Build history of the part. All positions in model axes, mm. A direction names the side the tool comes from. Give positions to 0.01 mm unless a question says otherwise; leave off trailing zeros. Order: outer loops, then holes, each group sorted by start corner. A loop starts at its lowest first (then second) coordinate and runs counter-clockwise, first axis right, second up. Notation, with made-up numbers: (37, 40.5) - (69, 40.5) arc R26 ccw to (69, 56.5) - close; hole circle Ø6 at (-35, 37.25). An arc over 180 degrees is marked (long way). Use a Markdown table: item, result. Add a question column.
(1) Slice it at C-C (z = -0.75). Write the cut outline in (x, y).
(2) Slice it at B-B (z = 5). Write the cut outline in (x, y) (1 decimal), then the cut area to 3 significant figures.
(3) Slice it at D-D (z = 13). Write the cut outline in (x, y).
(4) Flat gauge pins, fed straight in: pin 1 (0.9 mm diameter, centred on x = -23.5, y = 1.5, fed in from -Z); pin 2 (2.5 mm diameter, centred on y = 1, z = -2.5, fed in from -X). Where does each tip first touch, or does it go through?
(5) Which spindle directions (+Z, -Z, +X, -X, +Y, -Y) get a long thin tool onto all of the face, cutting with end or side? Do faces 4 (the face through (-23, 2, -5)), 5 (the face through (-26.873, 2.348, 4.918)), 6 (the face through (4.93, 2.41, 4.9)), 7 (the face through (23, 2, -5)), 8 (the face through (35, 2, 5)). Say none if no direction does.
(6) Slice it at A-A (y = 3.8). Write the cut outline in (x, z) (3 decimals), then the cut area to 3 significant figures.
(7) Wall check: line 1 (Z direction, x = 25, y = 3.1) (3 decimals); line 2 (X direction, y = 1.4, z = 5) (3 decimals); line 3 (Z direction, x = -23, y = 4.2). Give the ranges that are in metal, low to high.
(8) Mould opens along Z. For faces 1 (the face through (23.127, 2.348, 4.918)), 2 (the face through (-17.44, 2.41, -3.9)), 3 (the face through (0, 0, 11)) say: +Z half, -Z half, draft (parallel to the pull), parting line (faces both ways), or undercut.
from build123d import *

# Parameters (mm, degrees)
SKETCH1_R           = 1.875
BOSS_EXTRUDE1_DEPTH = 4.7625
CUT_EXTRUDE1_DEPTH  = 5.7625
BOSS_EXTRUDE2_DEPTH = 4.7625


with BuildPart() as part:
    # Sketch1 → Boss-Extrude1 (new body)
    with BuildSketch(Plane(origin=(0, 0, 0), x_dir=(1, 0, 0), z_dir=(0, 1, 0))):
        with BuildLine():
            Line((-25, 5), (25, 5))
            ThreePointArc((25, 5), (35, -5), (25, -15))
            Line((25, -15), (-25, -15))
            ThreePointArc((-25, -15), (-35, -5), (-25, 5))
        make_face()
        with Locations((-25, -5)):
            Circle(SKETCH1_R, mode=Mode.SUBTRACT)
        with Locations((25, -5)):
            Circle(SKETCH1_R, mode=Mode.SUBTRACT)
    extrude(amount=BOSS_EXTRUDE1_DEPTH)

    # Sketch3 → Cut-Extrude1 (cut, through all)
    with BuildSketch(Plane(origin=(0, 4.7625, 0), x_dir=(1, 0, 0), z_dir=(0, 1, 0))):
        with BuildLine():
            Line((-12.855000529, 3.026573405), (-1.414213562, -8.414213562))
            ThreePointArc((-1.414213562, -8.414213562), (0, -9), (1.414213562, -8.414213562))
            Line((1.414213562, -8.414213562), (12.855000529, 3.026573405))
            ThreePointArc((12.855000529, 3.026573405), (0, 164), (-12.855000529, 3.026573405))
        make_face()
    extrude(amount=-CUT_EXTRUDE1_DEPTH, mode=Mode.SUBTRACT)

    # Sketch4 → Boss-Extrude2 (add)
    with BuildSketch(Plane(origin=(0, 4.7625, 0), x_dir=(1, 0, 0), z_dir=(0, 1, 0))):
        with BuildLine():
            Line((14.377657426, 3.286243553), (8.551135427, -1.277291698))
            Line((8.551135427, -1.277291698), (8.551135427, 8.062765551))
            ThreePointArc((8.551135427, 8.062765551), (9.201135427, 8.712765551), (9.851135427, 8.062765551))
            Line((9.851135427, 8.062765551), (9.851135427, 7.812765551))
            Line((9.851135427, 7.812765551), (14.377657426, 3.286243553))
        make_face()
    extrude(amount=-BOSS_EXTRUDE2_DEPTH)


solid = part.part
Solution:
| question | item | result |
|---|---|---|
| 1 | outline | (-33.18, 0) - (-10.58, 0) - (-10.58, 4.76) - (-33.18, 4.76) - close; (8.55, 0) - (33.18, 0) - (33.18, 4.76) - (8.55, 4.76) - close |
| 2 | outline | (-35, 0) - (-26.9, 0) - (-26.9, 4.8) - (-35, 4.8) - close; (-23.1, 0) - (-4.8, 0) - (-4.8, 4.8) - (-23.1, 4.8) - close; (4.8, 0) - (23.1, 0) - (23.1, 4.8) - (4.8, 4.8) - close; (26.9, 0) - (35, 0) - (35, 4.8) - (26.9, 4.8) - close |
| 2 | area | 252 mm2 |
| 3 | outline | (-31, 0) - (31, 0) - (31, 4.76) - (-31, 4.76) - close |
| 4 | pin 1 | z = -5 |
| 4 | pin 2 | x = -32.81 |
| 5 | face 4 | -Z, -X, +Y, -Y |
| 5 | face 5 | +Y, -Y |
| 5 | face 6 | -Z, +Y, -Y |
| 5 | face 7 | -Z, +X, +Y, -Y |
| 5 | face 8 | +X, +Y, -Y |
| 6 | outline | (-25, -5) - (-21.84, -5) arc R81 cw to (-12.855, -3.027) - (-1.414, 8.414) arc R2 cw to (1.414, 8.414) - (8.551, 1.277) - (8.551, -8.063) arc R0.65 ccw to (9.851, -8.063) - (9.851, -7.813) - (14.378, -3.286) arc R81 cw to (21.84, -5) - (25, -5) arc R10 ccw to (25, 15) - (-25, 15) arc R10 ccw to start; hole circle Ø3.75 at (-25, 5); hole circle Ø3.75 at (25, 5) |
| 6 | area | 1,090 mm2 |
| 7 | line 1 | -5 to 3.125, 6.875 to 15 |
| 7 | line 2 | -35 to -26.875, -23.125 to -4.828, 4.828 to 23.125, 26.875 to 35 |
| 7 | line 3 | -5 to 15 |
| 8 | face 1 | undercut |
| 8 | face 2 | -Z half |
| 8 | face 3 | draft |
